CAD build for the part. Positions are in the model's coordinates, mm. A direction names the side the tool comes from. Coordinates: 2 decimals unless noted, no trailing zeros. Loops run counter-clockwise (first coordinate to the right, second up) from the corner with the lowest first, then second, coordinate; pieces in that order, holes last. Notation, with made-up numbers: (44.5, 15.5) -> (89.5, 15.5) arc R35 ccw to (89.5, 51.5) -> close; hole circle Ø11 at (60, 47.25). An arc over 180 degrees is marked (long way). Answer as CSV lines item,"result". Start each with the question number.
```python
from build123d import *

# Parameters (mm, degrees)
SKETCH1_W           = 25.4
SKETCH1_H           = 50.8
SKETCH1_W_2         = 19.05
SKETCH1_H_2         = 44.45
BOSS_EXTRUDE1_DEPTH = 63.5
SKETCH3_R           = 3.72872
SKETCH3_R_2         = 2.5527
CUT_EXTRUDE1_DEPTH  = 73.955945611


with BuildPart() as part:
    # Sketch1 → Boss-Extrude1 (new, symmetric)
    with BuildSketch(Plane.XY):
        Rectangle(SKETCH1_W, SKETCH1_H)
        Rectangle(SKETCH1_W_2, SKETCH1_H_2, mode=Mode.SUBTRACT)
    extrude(amount=BOSS_EXTRUDE1_DEPTH, both=True)

    # Sketch3 → Cut-Extrude1 (cut, through all)
    with BuildSketch(Plane(origin=(12.7, 0, 0), x_dir=(0, 0, -1), z_dir=(1, 0, 0))):
        with Locations(Location((50.8, -14.2875, 0), (0, 0, 90))):
            Circle(SKETCH3_R)
        with Locations(Location((-22.225, -14.2875, 0), (0, 0, 90))):
            Circle(SKETCH3_R)
        with Locations(Location((44.45, 14.2875, 0), (0, 0, 90))):
            Circle(SKETCH3_R_2)
        with Locations(Location((-15.875, 14.2875, 0), (0, 0, 90))):
            Circle(SKETCH3_R_2)
    extrude(amount=-CUT_EXTRUDE1_DEPTH, mode=Mode.SUBTRACT)


solid = part.part
```
Q1. Saw through at D-D (z = 11). List the corners of the cut face in (x, y) (3 decimals).
Q2. Probe probe 1 along X at (y, z) = (-21, -51) (3 decimals); probe 2 along Y at (x, z) = (4.5, 39) (3 decimals). List the from-to ranges inside material, lowest first. Write a range as from..to.
Q3. Saw through at C-C (x = -8). List the corners of the cut face in (y, z) (3 decimals), and give its area (3 significant figures).
Q4. Saw through at B-B (z = -50.8). List the corners of the cut face in (x, y) (3 decimals), and give its area (3 significant figures).
Q5. Which spindle directions (+Z, -Z, +X, -X, +Y, -Y) get a long thin tool onto all of the face, cutting with end or side? Do faces 1 (the flat face through (0, 22.225, 1)), 2 (the flat face through (0, -25.4, 1)). Say none if no direction does.
Q6. Saw through at A-A (y = 4). List the corners of the cut face in (x, z) (3 decimals).
Q7. Pin check, flat tip, straight feed: pin 1 Ø4 at (x, y) = (-8.5, 4.5) entering from +Z. Stop position of the tip, or through.
Q8. Two-plate mould, pull along Z, no slides. Class faces 3 (the cylindrical face through (-11.09, -15.096, 18.585)), 4 (the flat face through (-10, -2, -63.5)), 5 (the flat face through (0, 25.4, 1)): pulls with the +Z half, pulls with the -Z half, needs draft (parallel to the pull), parting line crosses it, or undercut.
Ans:
1,outline,"(-12.7, -25.4) -> (12.7, -25.4) -> (12.7, 25.4) -> (-12.7, 25.4) -> close; hole (-9.525, -22.225) -> (9.525, -22.225) -> (9.525, 22.225) -> (-9.525, 22.225) -> close"
2,probe 1,"x = -12.7..-9.525, 9.525..12.7"
2,probe 2,"y = -25.4..-22.225, 22.225..25.4"
3,outline,"(-25.4, -63.5) -> (-22.225, -63.5) -> (-22.225, 63.5) -> (-25.4, 63.5) -> close; (22.225, -63.5) -> (25.4, -63.5) -> (25.4, 63.5) -> (22.225, 63.5) -> close"
3,area,"806 mm²"
4,outline,"(-12.7, -25.4) -> (12.7, -25.4) -> (12.7, -18.016) -> (9.525, -18.016) -> (9.525, -22.225) -> (-9.525, -22.225) -> (-9.525, -18.016) -> (-12.7, -18.016) -> close; (-12.7, -10.559) -> (-9.525, -10.559) -> (-9.525, 22.225) -> (9.525, 22.225) -> (9.525, -10.559) -> (12.7, -10.559) -> (12.7, 25.4) -> (-12.7, 25.4) -> close"
4,area,"396 mm²"
5,face 1,"+Z, -Z"
5,face 2,"+Z, -Z, +X, -X, -Y"
6,outline,"(-12.7, -63.5) -> (-9.525, -63.5) -> (-9.525, 63.5) -> (-12.7, 63.5) -> close; (9.525, -63.5) -> (12.7, -63.5) -> (12.7, 63.5) -> (9.525, 63.5) -> close"
7,pin 1,"stops at z = 63.5"
8,face 3,"undercut"
8,face 4,"pulls with the -Z half"
8,face 5,"needs draft"
